Work out the finished part from the listing and answer in its coordinate system (mm). Face numbers are marked on the shaded views. Give positions to 0.01 mm unless a question says otherwise; leave off trailing zeros. Order: outer loops, then holes, each group sorted by start corner. A loop starts at its lowest first (then second) coordinate and runs counter-clockwise, first axis right, second up.
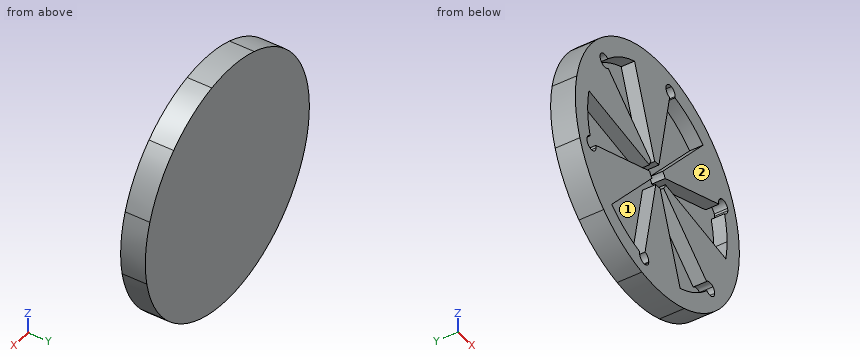
```python
from build123d import *

# Parameters (mm, degrees)
F1_DEPTH = 12.7
F2_R     = 63.5
F3_DEPTH = 5.842


# Not quite as in the source:
# - a feature names something its author has since deleted; it is built from what else it names


with BuildPart() as f1:
    # F0 (on Front) → F1 (new body)
    with BuildSketch(Plane.XZ):
        with BuildLine():
            Line((54.3616852417, 18.8314401648), (60.0018600902, 20.785254045))
            ThreePointArc((60.0018600902, 20.785254045), (52.5777266824, 35.6066378209), (41.57050809, 48.0014880722))
            Line((41.57050809, 48.0014880722), (35.3349318765, 40.8012648613))
            ThreePointArc((35.3349318765, 40.8012648613), (43.6698276291, 31.7213930943), (49.7275527638, 20.9874038681))
            ThreePointArc((49.7275527638, 20.9874038681), (52.5015720726, 20.8916190072), (54.3616852417, 18.8314401648))
        make_face()
        with BuildLine():
            Line((35.3349318765, 40.8012648613), (41.57050809, 48.0014880722))
            ThreePointArc((41.57050809, 48.0014880722), (27.7303280697, 57.1251162375), (12.000372018, 62.3557621349))
            Line((12.000372018, 62.3557621349), (10.8723370483, 56.4943204943))
            ThreePointArc((10.8723370483, 56.4943204943), (12.9421077904, 55.2668436539), (13.7563162153, 53.0023978147))
            ThreePointArc((13.7563162153, 53.0023978147), (13.7342201731, 52.6065963274), (13.6682066443, 52.2157136514))
            ThreePointArc((13.6682066443, 52.2157136514), (25.1574900679, 47.7535477057), (35.3349318765, 40.8012648613))
        make_face()
        with BuildLine():
            Line((10.8723370483, 56.4943204943), (12.000372018, 62.3557621349))
            ThreePointArc((12.000372018, 62.3557621349), (-4.5473895551, 63.3369658907), (-20.785254045, 60.0018600902))
            Line((-20.785254045, 60.0018600902), (-17.6674659382, 51.0015810767))
            ThreePointArc((-17.6674659382, 51.0015810767), (-5.6366184485, 53.6798766529), (6.6881514727, 53.5590258955))
            ThreePointArc((6.6881514727, 53.5590258955), (8.1581132499, 55.9135046571), (10.8723370483, 56.4943204943))
        make_face()
        with BuildLine():
            Line((-17.6674659382, 51.0015810767), (-20.785254045, 60.0018600902))
            ThreePointArc((-20.785254045, 60.0018600902), (-35.6066378209, 52.5777266824), (-48.0014880722, 41.57050809))
            Line((-48.0014880722, 41.57050809), (-43.4893481934, 37.6628803295))
            ThreePointArc((-43.4893481934, 37.6628803295), (-40.9974571589, 38.8855155725), (-38.3860311767, 37.9448710039))
            ThreePointArc((-38.3860311767, 37.9448710039), (-28.7770404, 45.6637993471), (-17.6674659382, 51.0015810767))
        make_face()
        with BuildLine():
            Line((-43.4893481934, 37.6628803295), (-48.0014880722, 41.57050809))
            ThreePointArc((-48.0014880722, 41.57050809), (-57.1251162375, 27.7303280697), (-62.3557621349, 12.000372018))
            Line((-62.3557621349, 12.000372018), (-53.0023978147, 10.2003162153))
            ThreePointArc((-53.0023978147, 10.2003162153), (-49.3064460776, 21.9584835586), (-43.0394012911, 32.5716220275))
            ThreePointArc((-43.0394012911, 32.5716220275), (-44.3434588227, 35.0218856499), (-43.4893481934, 37.6628803295))
        make_face()
        with BuildLine():
            Line((-53.0023978147, 10.2003162153), (-62.3557621349, 12.000372018))
            ThreePointArc((-62.3557621349, 12.000372018), (-63.3369658907, -4.5473895551), (-60.0018600902, -20.785254045))
            Line((-60.0018600902, -20.785254045), (-54.3616852417, -18.8314401648))
            ThreePointArc((-54.3616852417, -18.8314401648), (-54.1745729045, -16.062081604), (-52.054237821, -14.2708426476))
            ThreePointArc((-52.054237821, -14.2708426476), (-53.9345304679, -2.0897483586), (-53.0023978147, 10.2003162153))
        make_face()
        with BuildLine():
            ThreePointArc((-60.0018600902, -20.785254045), (-52.5777266824, -35.6066378209), (-41.57050809, -48.0014880722))
            Line((-41.57050809, -48.0014880722), (-35.3349318765, -40.8012648613))
            ThreePointArc((-35.3349318765, -40.8012648613), (-43.6698276292, -31.7213930943), (-49.7275527638, -20.9874038681))
            ThreePointArc((-49.7275527638, -20.9874038681), (-52.5015720726, -20.8916190072), (-54.3616852417, -18.8314401648))
            Line((-54.3616852417, -18.8314401648), (-60.0018600902, -20.785254045))
        make_face()
        with BuildLine():
            ThreePointArc((-41.57050809, -48.0014880722), (-27.7303280697, -57.1251162375), (-12.000372018, -62.3557621349))
            Line((-12.000372018, -62.3557621349), (-10.8723370483, -56.4943204943))
            ThreePointArc((-10.8723370483, -56.4943204943), (-13.1771157456, -54.9475971764), (-13.6682066443, -52.2157136514))
            ThreePointArc((-13.6682066443, -52.2157136514), (-25.1574900679, -47.7535477057), (-35.3349318765, -40.8012648613))
            Line((-35.3349318765, -40.8012648613), (-41.57050809, -48.0014880722))
        make_face()
        with BuildLine():
            ThreePointArc((-12.000372018, -62.3557621349), (4.5473895551, -63.3369658907), (20.785254045, -60.0018600902))
            Line((20.785254045, -60.0018600902), (17.6674659382, -51.0015810767))
            ThreePointArc((17.6674659382, -51.0015810767), (5.6366184485, -53.6798766529), (-6.6881514727, -53.5590258955))
            ThreePointArc((-6.6881514727, -53.5590258955), (-8.1581132499, -55.9135046571), (-10.8723370483, -56.4943204943))
            Line((-10.8723370483, -56.4943204943), (-12.000372018, -62.3557621349))
        make_face()
        with BuildLine():
            ThreePointArc((20.785254045, -60.0018600902), (35.6066378209, -52.5777266824), (48.0014880722, -41.57050809))
            Line((48.0014880722, -41.57050809), (43.4893481934, -37.6628803295))
            ThreePointArc((43.4893481934, -37.6628803295), (40.9974571589, -38.8855155725), (38.3860311767, -37.9448710039))
            ThreePointArc((38.3860311767, -37.9448710039), (28.7770404, -45.6637993471), (17.6674659382, -51.0015810767))
            Line((17.6674659382, -51.0015810767), (20.785254045, -60.0018600902))
        make_face()
        with BuildLine():
            ThreePointArc((48.0014880722, -41.57050809), (57.1251162375, -27.7303280697), (62.3557621349, -12.000372018))
            Line((62.3557621349, -12.000372018), (53.0023978147, -10.2003162153))
            ThreePointArc((53.0023978147, -10.2003162153), (49.3064460776, -21.9584835586), (43.0394012911, -32.5716220275))
            ThreePointArc((43.0394012911, -32.5716220275), (44.0109337807, -33.8041930262), (44.3572648613, -35.3349318765))
            ThreePointArc((44.3572648613, -35.3349318765), (44.1332282712, -36.5771701127), (43.4893481934, -37.6628803295))
            Line((43.4893481934, -37.6628803295), (48.0014880722, -41.57050809))
        make_face()
        with BuildLine():
            ThreePointArc((62.3557621349, -12.000372018), (63.2132932838, -6.0274001208), (63.5, 0))
            ThreePointArc((63.5, 0), (62.6193584913, 10.5387827635), (60.0018600902, 20.785254045))
            Line((60.0018600902, 20.785254045), (54.3616852417, 18.8314401648))
            ThreePointArc((54.3616852417, 18.8314401648), (54.5082651522, 18.257637773), (54.5575810767, 17.6674659382))
            ThreePointArc((54.5575810767, 17.6674659382), (53.864130935, 15.5577398165), (52.054237821, 14.2708426476))
            ThreePointArc((52.054237821, 14.2708426476), (53.4926542218, 7.1997617534), (53.975, 0))
            ThreePointArc((53.975, 0), (53.7312992912, -5.1232901027), (53.0023978147, -10.2003162153))
            Line((53.0023978147, -10.2003162153), (62.3557621349, -12.000372018))
        make_face()
        with BuildLine():
            ThreePointArc((-6.2355762135, 1.2000372018), (-5.7125116237, 2.773032807), (-4.8001488072, 4.157050809))
            Line((-4.8001488072, 4.157050809), (-38.1131815293, 33.0069834234))
            ThreePointArc((-38.1131815293, 33.0069834234), (-40.4882186348, 31.7927379151), (-43.0394012911, 32.5716220275))
            ThreePointArc((-43.0394012911, 32.5716220275), (-49.3064460776, 21.9584835586), (-53.0023978147, 10.2003162153))
            Line((-53.0023978147, 10.2003162153), (-6.2355762135, 1.2000372018))
        make_face()
        with BuildLine():
            ThreePointArc((-6.6881514727, -53.5590258955), (5.6366184485, -53.6798766529), (17.6674659382, -51.0015810767))
            Line((17.6674659382, -51.0015810767), (2.0785254045, -6.000186009))
            ThreePointArc((2.0785254045, -6.000186009), (0.4547389555, -6.3336965891), (-1.2000372018, -6.2355762135))
            Line((-1.2000372018, -6.2355762135), (-9.5282953823, -49.5104751351))
            ThreePointArc((-9.5282953823, -49.5104751351), (-7.4585246403, -50.7379519754), (-6.6443162153, -53.0023978147))
            ThreePointArc((-6.6443162153, -53.0023978147), (-6.6552919682, -53.2815735435), (-6.6881514727, -53.5590258955))
        make_face()
        with BuildLine():
            Line((-35.3349318765, -40.8012648613), (-4.157050809, -4.8001488072))
            ThreePointArc((-4.157050809, -4.8001488072), (-5.2577726682, -3.5606637821), (-6.000186009, -2.0785254045))
            Line((-6.000186009, -2.0785254045), (-47.6414769116, -16.5034917117))
            ThreePointArc((-47.6414769116, -16.5034917117), (-47.4948970012, -17.0772941035), (-47.4455810767, -17.6674659382))
            ThreePointArc((-47.4455810767, -17.6674659382), (-48.0710878861, -19.681751335), (-49.7275527638, -20.9874038681))
            ThreePointArc((-49.7275527638, -20.9874038681), (-43.6698276292, -31.7213930943), (-35.3349318765, -40.8012648613))
        make_face()
        with BuildLine():
            ThreePointArc((6.6881514727, 53.5590258955), (-5.6366184485, 53.6798766529), (-17.6674659382, 51.0015810767))
            Line((-17.6674659382, 51.0015810767), (-2.0785254045, 6.000186009))
            ThreePointArc((-2.0785254045, 6.000186009), (-0.4547389555, 6.3336965891), (1.2000372018, 6.2355762135))
            Line((1.2000372018, 6.2355762135), (9.5282953823, 49.5104751351))
            ThreePointArc((9.5282953823, 49.5104751351), (7.2892093729, 50.9601948492), (6.6881514727, 53.5590258955))
        make_face()
        with BuildLine():
            ThreePointArc((43.0394012911, -32.5716220275), (49.3064460776, -21.9584835586), (53.0023978147, -10.2003162153))
            Line((53.0023978147, -10.2003162153), (6.2355762135, -1.2000372018))
            ThreePointArc((6.2355762135, -1.2000372018), (5.7125116237, -2.773032807), (4.8001488072, -4.157050809))
            Line((4.8001488072, -4.157050809), (38.1131815293, -33.0069834234))
            ThreePointArc((38.1131815293, -33.0069834234), (40.4882186348, -31.7927379151), (43.0394012911, -32.5716220275))
        make_face()
        with BuildLine():
            ThreePointArc((49.7275527638, 20.9874038681), (43.6698276291, 31.7213930943), (35.3349318765, 40.8012648613))
            Line((35.3349318765, 40.8012648613), (4.157050809, 4.8001488072))
            ThreePointArc((4.157050809, 4.8001488072), (5.2577726682, 3.5606637821), (6.000186009, 2.0785254045))
            Line((6.000186009, 2.0785254045), (47.6414769116, 16.5034917117))
            ThreePointArc((47.6414769116, 16.5034917117), (47.7774280077, 19.1674569341), (49.7275527638, 20.9874038681))
        make_face()
    extrude(amount=F1_DEPTH)

    # F2 (on Front) → F3 (join)
    with BuildSketch(Plane.XZ):
        Circle(F2_R)
    extrude(amount=F3_DEPTH)


solid = f1.part
```
1. The mould has two halves that part along X. Classify the marked faces 1 and 2: pulls with the +X half, pulls with the -X half, needs draft (parallel to the pull), parting line crosses it, or undercut.
Findings below:
face 1: undercut
face 2: needs draft
2. The part is cut by section B-B (x = 24.5). Write down the section's boundary in (y, z).
Findings below:
outline: (-12.7, -58.58) - (0, -58.58) - (0, 58.58) - (-12.7, 58.58) - (-12.7, 48.09) - (-5.84, 48.09) - (-5.84, 28.29) - (-12.7, 28.29) - (-12.7, 8.49) - (-5.84, 8.49) - (-5.84, -4.72) - (-12.7, -4.72) - (-12.7, -21.22) - (-5.84, -21.22) - (-5.84, -48.09) - (-12.7, -48.09) - close
3. Given P1, Ø3, axis at y = -2.5, z = 50, coming from the +X side; P2, Ø1, axis at x = -34.5, y = -6.5, coming from the +Z side; P3, Ø2, axis at y = -3.5, z = -31, coming from the -X side; P4, Ø1, axis at x = 14.5, z = 50.5, coming from the +Y side, each flat-ended and moving along its own axis, determine where each tip first touches the part or whether it passes through.
Findings below:
P1: stops at x = 40.99
P2: stops at z = 53.63
P3: stops at x = -55.97
P4: stops at y = 0
4. The part is cut by section C-C (z = 43.5). Write down the section's boundary in (x, y).
Findings below:
outline: (-46.26, -12.7) - (-31.95, -12.7) - (-31.95, -5.84) - (-15.07, -5.84) - (-15.07, -12.7) - (8.37, -12.7) - (8.37, -5.84) - (31.95, -5.84) - (31.95, -12.7) - (46.26, -12.7) - (46.26, 0) - (-46.26, 0) - close
5. Straight lines are drawn through the part: probe 1 along X at (y, z) = (-10.5, -49); probe 2 along Z at (x, y) = (-30.5, -7); probe 3 along X at (y, z) = (-7.25, 47.5). For each, find the intervals that lie inside material, in ascending order.
Findings below:
probe 1: x = -40.39 to -22.63, -9.43 to 16.97, 22.63 to 40.39
probe 2: z = -55.7 to -44.53, -35.22 to -10.57, 5.87 to 26.41, 44.53 to 55.7
probe 3: x = -42.14 to -25.63, -16.45 to 9.14, 25.63 to 42.14
6. The part is cut by section A-A (y = -3). Write down the section's boundary in (x, z).
Findings below:
outline: circle Ø127 at (0, 0)
